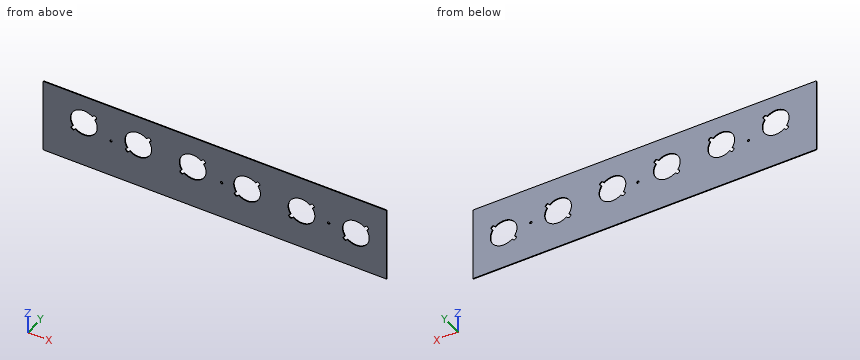
```python
from build123d import *

# Parameters (mm, degrees)
SKETCH2_W             = 635
SKETCH2_H             = 139.7
BOSS_EXTRUDE1_DEPTH   = 1.524
FILLET1_R             = 1.27
F_8_CLEARANCE_HOLE1_D = 4.3053


with BuildPart() as part:
    # Sketch2 → Boss-Extrude1 (new body)
    with BuildSketch(Plane(origin=(0, 0, 0), x_dir=(1, 0, 0), z_dir=(0, 1, 0))):
        Rectangle(SKETCH2_W, SKETCH2_H)
        with BuildLine():
            Line((180.471121526, -17.560883985), (183.417760323, -20.322450333))
            ThreePointArc((183.417760323, -20.322450333), (184.049066919, -21.716938673), (183.509415933, -23.14939201))
            Line((183.509415933, -23.14939201), (181.663097836, -25.119445179))
            ThreePointArc((181.663097836, -25.119445179), (180.268609495, -25.750751775), (178.836156158, -25.211100788))
            Line((178.836156158, -25.211100788), (175.889517361, -22.44953444))
            ThreePointArc((175.889517361, -22.44953444), (143.413950131, -21.293785193), (140.156982214, 11.038712132))
            Line((140.156982214, 11.038712132), (137.210343417, 13.80027848))
            ThreePointArc((137.210343417, 13.80027848), (136.579036821, 15.194766821), (137.118687808, 16.627220158))
            Line((137.118687808, 16.627220158), (138.965005904, 18.597273327))
            ThreePointArc((138.965005904, 18.597273327), (140.359494245, 19.228579923), (141.791947582, 18.688928936))
            Line((141.791947582, 18.688928936), (144.738586379, 15.927362588))
            ThreePointArc((144.738586379, 15.927362588), (177.214153609, 14.77161334), (180.471121526, -17.560883985))
        make_face(mode=Mode.SUBTRACT)
        with BuildLine():
            Line((242.373895712, 21.950014862), (245.320534509, 19.188448514))
            ThreePointArc((245.320534509, 19.188448514), (277.796101739, 18.032699267), (281.053069656, -14.299798058))
            Line((281.053069656, -14.299798058), (283.999708453, -17.061364407))
            ThreePointArc((283.999708453, -17.061364407), (284.631015049, -18.455852747), (284.091364062, -19.888306084))
            Line((284.091364062, -19.888306084), (282.245045966, -21.858359253))
            ThreePointArc((282.245045966, -21.858359253), (280.850557625, -22.489665849), (279.418104288, -21.950014862))
            Line((279.418104288, -21.950014862), (276.471465491, -19.188448514))
            ThreePointArc((276.471465491, -19.188448514), (243.995898261, -18.032699267), (240.738930344, 14.299798058))
            Line((240.738930344, 14.299798058), (237.792291547, 17.061364407))
            ThreePointArc((237.792291547, 17.061364407), (237.160984951, 18.455852747), (237.700635938, 19.888306084))
            Line((237.700635938, 19.888306084), (239.546954034, 21.858359253))
            ThreePointArc((239.546954034, 21.858359253), (240.941442375, 22.489665849), (242.373895712, 21.950014862))
        make_face(mode=Mode.SUBTRACT)
        with BuildLine():
            Line((39.575034084, 7.777626206), (36.628395287, 10.539192554))
            ThreePointArc((36.628395287, 10.539192554), (35.997088691, 11.933680895), (36.536739678, 13.366134232))
            Line((36.536739678, 13.366134232), (38.383057774, 15.336187401))
            ThreePointArc((38.383057774, 15.336187401), (39.777546115, 15.967493997), (41.209999452, 15.42784301))
            Line((41.209999452, 15.42784301), (44.156638249, 12.666276662))
            ThreePointArc((44.156638249, 12.666276662), (76.632205479, 11.510527414), (79.889173396, -20.821969911))
            Line((79.889173396, -20.821969911), (82.835812193, -23.583536259))
            ThreePointArc((82.835812193, -23.583536259), (83.467118789, -24.9780246), (82.927467803, -26.410477937))
            Line((82.927467803, -26.410477937), (81.081149706, -28.380531105))
            ThreePointArc((81.081149706, -28.380531105), (79.686661366, -29.011837701), (78.254208028, -28.472186714))
            Line((78.254208028, -28.472186714), (75.307569231, -25.710620366))
            ThreePointArc((75.307569231, -25.710620366), (42.832002001, -24.554871119), (39.575034084, 7.777626206))
        make_face(mode=Mode.SUBTRACT)
        with BuildLine():
            Line((-61.006914046, 4.51654028), (-63.953552843, 7.278106628))
            ThreePointArc((-63.953552843, 7.278106628), (-64.584859439, 8.672594969), (-64.045208452, 10.105048306))
            Line((-64.045208452, 10.105048306), (-62.198890356, 12.075101475))
            ThreePointArc((-62.198890356, 12.075101475), (-60.804402015, 12.706408071), (-59.371948678, 12.166757084))
            Line((-59.371948678, 12.166757084), (-56.425309881, 9.405190735))
            ThreePointArc((-56.425309881, 9.405190735), (-23.949742651, 8.249441488), (-20.692774734, -24.083055837))
            Line((-20.692774734, -24.083055837), (-17.746135937, -26.844622185))
            ThreePointArc((-17.746135937, -26.844622185), (-17.114829341, -28.239110526), (-17.654480327, -29.671563863))
            Line((-17.654480327, -29.671563863), (-19.500798424, -31.641617031))
            ThreePointArc((-19.500798424, -31.641617031), (-20.895286764, -32.272923627), (-22.327740102, -31.73327264))
            Line((-22.327740102, -31.73327264), (-25.274378899, -28.971706292))
            ThreePointArc((-25.274378899, -28.971706292), (-57.749946129, -27.815957045), (-61.006914046, 4.51654028))
        make_face(mode=Mode.SUBTRACT)
        with BuildLine():
            Line((-161.588862176, 1.255454354), (-164.535500973, 4.017020702))
            ThreePointArc((-164.535500973, 4.017020702), (-165.166807569, 5.411509043), (-164.627156582, 6.84396238))
            Line((-164.627156582, 6.84396238), (-162.780838486, 8.814015548))
            ThreePointArc((-162.780838486, 8.814015548), (-161.386350145, 9.445322144), (-159.953896808, 8.905671157))
            Line((-159.953896808, 8.905671157), (-157.007258011, 6.144104809))
            ThreePointArc((-157.007258011, 6.144104809), (-124.53169078, 4.988355562), (-121.274722864, -27.344141763))
            Line((-121.274722864, -27.344141763), (-118.328084067, -30.105708111))
            ThreePointArc((-118.328084067, -30.105708111), (-117.696777471, -31.500196452), (-118.236428457, -32.932649789))
            Line((-118.236428457, -32.932649789), (-120.082746554, -34.902702958))
            ThreePointArc((-120.082746554, -34.902702958), (-121.477234894, -35.534009554), (-122.909688232, -34.994358567))
            Line((-122.909688232, -34.994358567), (-125.856327029, -32.232792218))
            ThreePointArc((-125.856327029, -32.232792218), (-158.331894259, -31.077042971), (-161.588862176, 1.255454354))
        make_face(mode=Mode.SUBTRACT)
        with BuildLine():
            Line((-221.856670994, -30.605227689), (-218.910032197, -33.366794037))
            ThreePointArc((-218.910032197, -33.366794037), (-218.2787256, -34.761282378), (-218.818376587, -36.193735715))
            Line((-218.818376587, -36.193735715), (-220.664694684, -38.163788884))
            ThreePointArc((-220.664694684, -38.163788884), (-222.059183024, -38.79509548), (-223.491636361, -38.255444493))
            Line((-223.491636361, -38.255444493), (-226.438275159, -35.493878145))
            ThreePointArc((-226.438275159, -35.493878145), (-258.913842389, -34.338128897), (-262.170810306, -2.005631572))
            Line((-262.170810306, -2.005631572), (-265.117449103, 0.755934776))
            ThreePointArc((-265.117449103, 0.755934776), (-265.748755699, 2.150423117), (-265.209104712, 3.582876454))
            Line((-265.209104712, 3.582876454), (-263.362786616, 5.552929622))
            ThreePointArc((-263.362786616, 5.552929622), (-261.968298275, 6.184236218), (-260.535844938, 5.644585231))
            Line((-260.535844938, 5.644585231), (-257.589206141, 2.883018883))
            ThreePointArc((-257.589206141, 2.883018883), (-225.11363891, 1.727269636), (-221.856670994, -30.605227689))
        make_face(mode=Mode.SUBTRACT)
    extrude(amount=BOSS_EXTRUDE1_DEPTH)

    # Fillet1
    fillet1_edges = [part.edges().sort_by_distance(p)[0] for p in [
        (-317.5, 0.762, 69.85),
        (-317.5, 0.762, -69.85),
    ]]
    fillet(fillet1_edges, radius=FILLET1_R)

    # #8 Clearance Hole1 (through all)
    with Locations(Plane(origin=(0, 1.524, 0), x_dir=(1, 0, 0), z_dir=(0, 1, 0))):
        with Locations((210.5786, 0), (12.7, 0), (-191.9606, 0)):
            Hole(F_8_CLEARANCE_HOLE1_D / 2)


solid = part.part
```
Design review of the part built by this model. Coordinates are the model's own, in mm. Coordinates: 2 decimals unless noted, no trailing zeros. Loops run counter-clockwise (first coordinate to the right, second up) from the corner with the lowest first, then second, coordinate; pieces in that order, holes last. Notation, with made-up numbers: (76.5, 36.25) -> (93.5, 36.25) arc R18 cw to (93.5, 46.25) -> close; hole circle Ø3 at (2.5, 56.5). An arc over 180 degrees is marked (long way). Answer as a JSON object with one key per item and string values.
Q1. To check wall thickness, follow L1, parallel to Z at x = 12.7, y = 0.8; L2, parallel to Z at x = 144, y = 0.8; L3, parallel to Z at x = -221.5, y = 1.25. State the ranges of each line that lie inside material, in increasing order.
Answer block:
{"L1": "z = -69.85 to -2.15, 2.15 to 69.85", "L2": "z = -69.85 to -16.62, 21.83 to 69.85", "L3": "z = -69.85 to 2.52, 30.09 to 30.94, 38.7 to 69.85"}
Q2. Take a section at B-B on y = 0.4. Give the number of separate pieces and of enclosed holes in the cut face, plus the area to 3 significant figures.
Answer block:
{"separate pieces": "1", "enclosed holes": "9", "area": "76,700 mm^2"}
Q3. Take a section at A-A on x = -233. Give the boundary of the cut face in (y, z), plus the area to 3 significant figures.
Answer block:
{"outline": "(0, -69.85) -> (1.52, -69.85) -> (1.52, -6.71) -> (0, -6.71) -> close; (0, 39.32) -> (1.52, 39.32) -> (1.52, 69.85) -> (0, 69.85) -> close", "area": "143 mm^2"}
